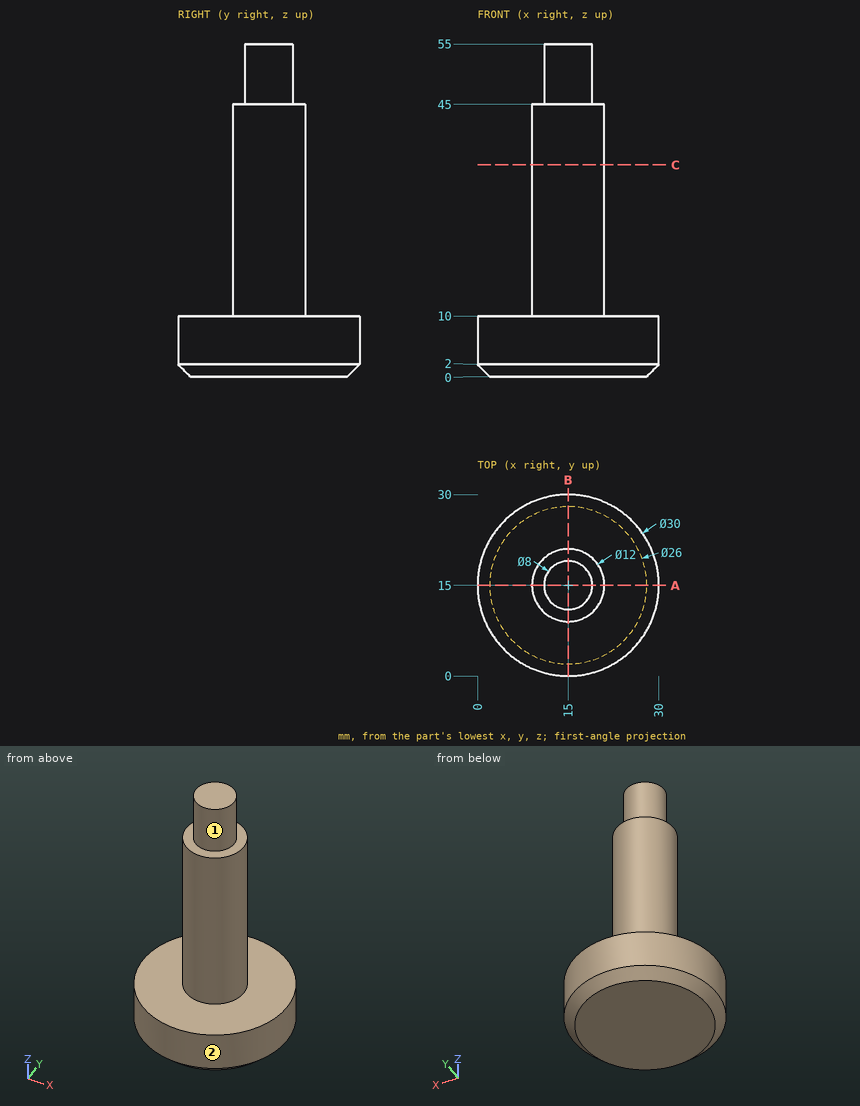
Can you work these out from the drawing? Everything is in mm from the part's minimum corner. A direction names the side the tool comes from. Coordinates: 2 decimals unless noted, no trailing zeros. Write each loop counter-clockwise with the first axis right and the second up, starting at its lowest first coordinate (ties: lowest second). Pieces come first, ordered by that corner, then holes. Notation, with made-up numbers: (59.25, -15) - (84.25, -15) arc R30 cw to (84.25, 19) - close; hole circle Ø5 at (45, 88). An arc over 180 degrees is marked (long way). One line per item, written item: value.
1) I'm going to push flat-ended pins straight in: P1, Ø2, axis at y = 19.5, z = 14, coming from the -X side; P2, Ø2, axis at x = 24, y = 9, coming from the +Z side. Where does each tip first touch, or does it pass through?
Model answer:
P1: stops at x = 10.13
P2: stops at z = 10
2) On a 3-axis mill with a long thin cutter (end or side, diameter ignored), from which of +Z, -Z, +X, -X, +Y, -Y can I reach the whole of each face in a straight line? I mean the marked faces 1 and 2. Say none if no direction works.
Model answer:
face 1: +Z
face 2: +Z, -Z
3) Suppose I cut it at A-A on y = 15. Write out the boundary of the cut face in (x, z), and give its area (3 significant figures).
Model answer:
outline: (0, 2) - (2, 0) - (28, 0) - (30, 2) - (30, 10) - (21, 10) - (21, 45) - (19, 45) - (19, 55) - (11, 55) - (11, 45) - (9, 45) - (9, 10) - (0, 10) - close
area: 796 mm²
4) I need wall thicknesses on line 1 along Z through (x, y) = (4.75, 22); line 2 along Y through (x, z) = (15.5, 8); line 3 along Y through (x, z) = (11.5, 26). Which ranges of each line are inside material? Lowest first, please.
Model answer:
line 1: z = 0 to 10
line 2: y = 0.01 to 29.99
line 3: y = 10.13 to 19.87
5) Suppose I cut it at C-C on z = 35. Write out the boundary of the cut face in (x, y), and give its area (3 significant figures).
Model answer:
outline: circle Ø12 at (15, 15)
area: 113 mm²
